```python
from build123d import *

# Parameters (mm, degrees)
SKETCH1_R               = 2.125
BOSS_EXTRUDE1_DEPTH     = 2
BOSS_EXTRUDE3_DEPTH     = 2
BOSS_EXTRUDE4_DEPTH     = 2
FILLET1_R               = 2.5
SKETCH6_R               = 2.025
CUT_EXTRUDE1_DEPTH      = 1
CUT_EXTRUDE1_DEPTH_BACK = 3


with BuildPart() as part:
    # Sketch1 → Boss-Extrude1 (new body)
    with BuildSketch(Plane(origin=(0, 0, 0), x_dir=(1, 0, 0), z_dir=(0, 1, 0))):
        with BuildLine():
            Line((-37.655823606, 28.125414637), (-49.673639651, 37.101610798))
            ThreePointArc((-49.673639651, 37.101610798), (-59.88740123, 16.046780796), (-61.569439235, -7.294117647))
            Line((-61.569439235, -7.294117647), (-46.673607162, -5.529411765))
            ThreePointArc((-46.673607162, -5.529411765), (-45.398513836, 12.16449512), (-37.655823606, 28.125414637))
        make_face()
        with Locations((-44.167295593, 25.5)):
            Circle(SKETCH1_R, mode=Mode.SUBTRACT)
        with Locations((-51.095498823, 29.5)):
            Circle(SKETCH1_R, mode=Mode.SUBTRACT)
        with Locations((-59, 0)):
            Circle(SKETCH1_R, mode=Mode.SUBTRACT)
        with Locations((-51, 0)):
            Circle(SKETCH1_R, mode=Mode.SUBTRACT)
    extrude(amount=BOSS_EXTRUDE1_DEPTH)

    # Sketch3 → Boss-Extrude3 (add)
    with BuildSketch(Plane(origin=(0, 0, 0), x_dir=(1, 0, 0), z_dir=(0, 1, 0))):
        with BuildLine():
            Line((-62.506368953, 35.734490906), (-53.824928821, 30.771367169))
            ThreePointArc((-53.824928821, 30.771367169), (-51.845987454, 33.999905661), (-49.673639651, 37.101610798))
            Line((-49.673639651, 37.101610798), (-57.685517014, 43.085741572))
            ThreePointArc((-57.685517014, 43.085741572), (-60.208243494, 39.483761413), (-62.506368953, 35.734490906))
        make_face()
    extrude(amount=BOSS_EXTRUDE3_DEPTH)

    # Sketch5 → Boss-Extrude4 (add)
    with BuildSketch(Plane(origin=(0, 0, 0), x_dir=(1, 0, 0), z_dir=(0, 1, 0))):
        with BuildLine():
            Line((-47.466920684, 54.137708123), (-40.874292811, 46.618581995))
            ThreePointArc((-40.874292811, 46.618581995), (-45.523347894, 42.09067351), (-49.673639651, 37.101610798))
            Line((-49.673639651, 37.101610798), (-57.685517014, 43.085741572))
            ThreePointArc((-57.685517014, 43.085741572), (-52.865823361, 48.879491818), (-47.466920684, 54.137708123))
        make_face()
    extrude(amount=BOSS_EXTRUDE4_DEPTH)

    # Fillet1
    fillet1_edges = [part.edges().sort_by_distance(p)[0] for p in [
        (-53.824928821, 1, -30.771367169),
        (-62.506368953, 1, -35.734490906),
        (-49.673639651, 1, -37.101610798),
        (-46.673607162, 1, 5.529411765),
        (-61.569439235, 1, 7.294117647),
        (-37.655823606, 1, -28.125414637),
    ]]
    fillet(fillet1_edges, radius=FILLET1_R)

    # Sketch6 → Cut-Extrude1 (cut, two sides)
    with BuildSketch(Plane(origin=(0, 2, 0), x_dir=(1, 0, 0), z_dir=(0, 1, 0))) as cut_extrude1_sk:
        with Locations((-46.746660862, 47.99739262)):
            Circle(SKETCH6_R)
    extrude(amount=CUT_EXTRUDE1_DEPTH, mode=Mode.SUBTRACT)
    extrude(cut_extrude1_sk.sketch, amount=-CUT_EXTRUDE1_DEPTH_BACK, mode=Mode.SUBTRACT)


solid = part.part
```
Check sheet for the modelled part. Datum: model origin and axes. Units: mm. A direction names the side the tool comes from. Round coordinates to 2 decimals unless told otherwise and drop trailing zeros. Order: outer loops, then holes, each group sorted by start corner. A loop starts at its lowest first (then second) coordinate and runs counter-clockwise, first axis right, second up.
1) Mould release check, pull along Z, two halves, no side actions. Record for faces 1 (the flat face through (-44.217, 0.986, -50.431)), 2 (the flat face through (-53, 0, -24)), 3 (the cylindrical face through (-60.939, 1.014, 6.424)), 4 (the cylindrical face through (-60.686, 0.986, -12.696)): +Z half, -Z half, draft (parallel to the pull), parting line (faces both ways), or undercut.
2) Go/stop test with a flat-tipped pin: pin 1 Ø7 at (x, z) = (-51, 0) entering from +Y. Record where the tip stops, or that it passes through.
3) Tool access check on faces 5 (the cylindrical face through (-52.782, 0.986, -28.207)), 6 (the flat face through (-58.16, 0.99, -33.25)), 7 (the cylindrical face through (-44.58, 0.99, -43.09)). Record the directions out of +Z, -Z, +X, -X, +Y, -Y that give a thin tool (end or side, any length) a straight path to the whole face; none if there is none.
4) Section check D-D (y = 0.8). Give the number of separate pieces and of enclosed holes in the cut face, and give its area (3 significant figures).
5) Scan lines: line 1 (X direction, y = 0.7, z = 0) (3 decimals); line 2 (Z direction, x = -52.75, y = 1.4); line 3 (Z direction, x = -52, y = 0.6) (3 decimals). Record each from-to range of solid material in increasing order.
6) Section check B-B (x = -51). Record the boundary of the cut face in (y, z) (3 decimals), and give its area (3 significant figures).
7) Section check A-A (z = 0). Record the boundary of the cut face in (x, y) (3 decimals), and give its area (3 significant figures).
8) Section check C-C (z = -25.5). Record the boundary of the cut face in (x, y).
Result:
1. face 1: -Z half
1. face 2: draft
1. face 3: +Z half
1. face 4: undercut
2. pin 1: stops at y = 2
3. face 5: +Y, -Y
3. face 6: -X, +Y, -Y
3. face 7: +X, +Y, -Y
4. separate pieces: 1
4. enclosed holes: 5
4. area: 771 mm2
5. line 1: x = -62 to -61.125, -56.875 to -53.125, -48.875 to -47
5. line 2: z = -49 to -30.83, -28.17 to -1.21, 1.21 to 6.25
5. line 3: z = -49.8 to -31.423, -27.577 to -1.875, 1.875 to 6.16
6. outline: (0, -50.823) - (2, -50.823) - (2, -31.623) - (0, -31.623) - close; (0, -27.377) - (2, -27.377) - (2, -2.125) - (0, -2.125) - close; (0, 2.125) - (2, 2.125) - (2, 6.042) - (0, 6.042) - close
6. area: 96.7 mm2
7. outline: (-62, 0) - (-61.125, 0) - (-61.125, 2) - (-62, 2) - close; (-56.875, 0) - (-53.125, 0) - (-53.125, 2) - (-56.875, 2) - close; (-48.875, 0) - (-47, 0) - (-47, 2) - (-48.875, 2) - close
7. area: 13.0 mm2
8. outline: (-56.51, 0) - (-46.29, 0) - (-46.29, 2) - (-56.51, 2) - close; (-42.04, 0) - (-39.48, 0) - (-39.48, 2) - (-42.04, 2) - close
